Can you work these out from the drawing? Everything is in mm from the part's minimum corner. Give positions to 0.01 mm unless a question says otherwise; leave off trailing zeros. Order: outer loops, then holes, each group sorted by start corner. A loop starts at its lowest first (then second) coordinate and runs counter-clockwise, first axis right, second up. Notation, with made-up numbers: M 71.5,-26.75 L 101.5,-26.75 A21 ccw 101.5,1.25 Z; hole C 6.5,83.5 d3. An arc over 180 degrees is marked long. Answer in a Markdown table with one row per item. Add a question column.
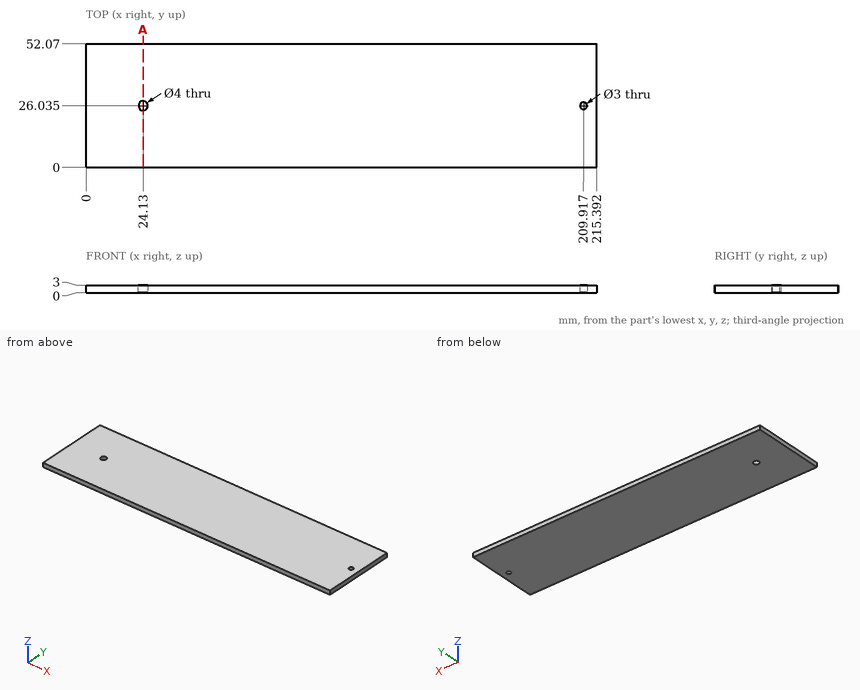
1. If I drill on line 1 along X through (y, z) = (26, 0.65); line 2 along Y through (x, z) = (24.13, 0.7) (1 decimal), over which ranges is the centre line in solid material (lowest first)? Write a range as [from, to].
2. Suppose I cut it at A-A on x = 24.13. List the corners of the cut face in (y, z) for me (1 decimal).
3. Will these pins go through, and if not, where does the flat tip stop? P1, Ø1.8, axis at x = 209.92, y = 26.04, coming from the +Z side; P2, Ø1.5, axis at x = 125, z = 2, coming from the -Y side.
Findings below:
| question | item | result |
|---|---|---|
| 1 | line 1 | [0, 22.13], [26.13, 208.42], [211.42, 215.39] |
| 1 | line 2 | [0, 24], [28, 52.1] |
| 2 | outline | M 0,0 L 24,0 L 24,3 L 0,3 Z; M 28,0 L 52.1,0 L 52.1,3 L 28,3 Z |
| 3 | P1 | through |
| 3 | P2 | y = 0 |
